from build123d import *

# Parameters (mm, degrees)
CUT_EXTRUDE_1_DEPTH = 8
SKETCH_7_R          = 4.1
CUT_EXTRUDE_3_DEPTH = 10


with BuildPart() as part:
    # 草图1 → 旋转1 (revolve)
    with BuildSketch(Plane.XY):
        Polygon((-9.5, 0), (9.5, 0), (9.5, 13), (8, 13), (8, 11.05), (-8, 11.05), (-8, 13), (-9.5, 13), align=None)
    revolve(axis=Axis((-9.5, 0, 0), (1, 0, 0)))

    # 草图2 → 切除-拉伸1 (cut, symmetric)
    with BuildSketch(Plane(origin=(0, 0, 0), x_dir=(0, 0, -1), z_dir=(1, 0, 0))):
        with BuildLine():
            Line((11.05, 0), (10, 0))
            ThreePointArc((10, 0), (9.969173337, 0.784590957), (9.876883406, 1.56434465))
            Line((9.876883406, 1.56434465), (10.913956164, 1.728600839))
            ThreePointArc((10.913956164, 1.728600839), (11.015936538, 0.866973008), (11.05, 0))
        make_face()
        with BuildLine():
            Line((10.509174505, -3.414637788), (9.510565163, -3.090169944))
            ThreePointArc((9.510565163, -3.090169944), (9.723699204, -2.334453639), (9.876883406, -1.56434465))
            Line((9.876883406, -1.56434465), (10.913956164, -1.728600839))
            ThreePointArc((10.913956164, -1.728600839), (10.74468762, -2.579571271), (10.509174505, -3.414637788))
        make_face()
        with BuildLine():
            Line((8.939637788, -6.495027038), (8.090169944, -5.877852523))
            ThreePointArc((8.090169944, -5.877852523), (8.526401644, -5.224985647), (8.910065242, -4.539904997))
            Line((8.910065242, -4.539904997), (9.845622092, -5.016595022))
            ThreePointArc((9.845622092, -5.016595022), (9.421673816, -5.77360914), (8.939637788, -6.495027038))
        make_face()
        with BuildLine():
            Line((6.495027038, -8.939637788), (5.877852523, -8.090169944))
            ThreePointArc((5.877852523, -8.090169944), (6.494480483, -7.604059656), (7.071067812, -7.071067812))
            Line((7.071067812, -7.071067812), (7.813529932, -7.813529932))
            ThreePointArc((7.813529932, -7.813529932), (7.176400934, -8.40248592), (6.495027038, -8.939637788))
        make_face()
        with BuildLine():
            Line((3.414637788, -10.509174505), (3.090169944, -9.510565163))
            ThreePointArc((3.090169944, -9.510565163), (3.826834324, -9.238795325), (4.539904997, -8.910065242))
            Line((4.539904997, -8.910065242), (5.016595022, -9.845622092))
            ThreePointArc((5.016595022, -9.845622092), (4.228651928, -10.208868834), (3.414637788, -10.509174505))
        make_face()
        with BuildLine():
            Line((0, -11.05), (0, -10))
            ThreePointArc((0, -10), (0.784590957, -9.969173337), (1.56434465, -9.876883406))
            Line((1.56434465, -9.876883406), (1.728600839, -10.913956164))
            ThreePointArc((1.728600839, -10.913956164), (0.866973008, -11.015936538), (0, -11.05))
        make_face()
        with BuildLine():
            Line((-3.414637788, -10.509174505), (-3.090169944, -9.510565163))
            ThreePointArc((-3.090169944, -9.510565163), (-2.334453639, -9.723699204), (-1.56434465, -9.876883406))
            Line((-1.56434465, -9.876883406), (-1.728600839, -10.913956164))
            ThreePointArc((-1.728600839, -10.913956164), (-2.579571271, -10.74468762), (-3.414637788, -10.509174505))
        make_face()
        with BuildLine():
            Line((-6.495027038, -8.939637788), (-5.877852523, -8.090169944))
            ThreePointArc((-5.877852523, -8.090169944), (-5.224985647, -8.526401644), (-4.539904997, -8.910065242))
            Line((-4.539904997, -8.910065242), (-5.016595022, -9.845622092))
            ThreePointArc((-5.016595022, -9.845622092), (-5.77360914, -9.421673816), (-6.495027038, -8.939637788))
        make_face()
        with BuildLine():
            Line((-8.939637788, -6.495027038), (-8.090169944, -5.877852523))
            ThreePointArc((-8.090169944, -5.877852523), (-7.604059656, -6.494480483), (-7.071067812, -7.071067812))
            Line((-7.071067812, -7.071067812), (-7.813529932, -7.813529932))
            ThreePointArc((-7.813529932, -7.813529932), (-8.40248592, -7.176400934), (-8.939637788, -6.495027038))
        make_face()
        with BuildLine():
            Line((-10.509174505, -3.414637788), (-9.510565163, -3.090169944))
            ThreePointArc((-9.510565163, -3.090169944), (-9.238795325, -3.826834324), (-8.910065242, -4.539904997))
            Line((-8.910065242, -4.539904997), (-9.845622092, -5.016595022))
            ThreePointArc((-9.845622092, -5.016595022), (-10.208868834, -4.228651928), (-10.509174505, -3.414637788))
        make_face()
        with BuildLine():
            Line((-11.05, 0), (-10, 0))
            ThreePointArc((-10, 0), (-9.969173337, -0.784590957), (-9.876883406, -1.56434465))
            Line((-9.876883406, -1.56434465), (-10.913956164, -1.728600839))
            ThreePointArc((-10.913956164, -1.728600839), (-11.015936538, -0.866973008), (-11.05, 0))
        make_face()
        with BuildLine():
            Line((-10.509174505, 3.414637788), (-9.510565163, 3.090169944))
            ThreePointArc((-9.510565163, 3.090169944), (-9.723699204, 2.334453639), (-9.876883406, 1.56434465))
            Line((-9.876883406, 1.56434465), (-10.913956164, 1.728600839))
            ThreePointArc((-10.913956164, 1.728600839), (-10.74468762, 2.579571271), (-10.509174505, 3.414637788))
        make_face()
        with BuildLine():
            Line((-8.939637788, 6.495027038), (-8.090169944, 5.877852523))
            ThreePointArc((-8.090169944, 5.877852523), (-8.526401644, 5.224985647), (-8.910065242, 4.539904997))
            Line((-8.910065242, 4.539904997), (-9.845622092, 5.016595022))
            ThreePointArc((-9.845622092, 5.016595022), (-9.421673816, 5.77360914), (-8.939637788, 6.495027038))
        make_face()
        with BuildLine():
            Line((-6.495027038, 8.939637788), (-5.877852523, 8.090169944))
            ThreePointArc((-5.877852523, 8.090169944), (-6.494480483, 7.604059656), (-7.071067812, 7.071067812))
            Line((-7.071067812, 7.071067812), (-7.813529932, 7.813529932))
            ThreePointArc((-7.813529932, 7.813529932), (-7.176400934, 8.40248592), (-6.495027038, 8.939637788))
        make_face()
        with BuildLine():
            Line((-3.414637788, 10.509174505), (-3.090169944, 9.510565163))
            ThreePointArc((-3.090169944, 9.510565163), (-3.826834324, 9.238795325), (-4.539904997, 8.910065242))
            Line((-4.539904997, 8.910065242), (-5.016595022, 9.845622092))
            ThreePointArc((-5.016595022, 9.845622092), (-4.228651928, 10.208868834), (-3.414637788, 10.509174505))
        make_face()
        with BuildLine():
            Line((0, 11.05), (0, 10))
            ThreePointArc((0, 10), (-0.784590957, 9.969173337), (-1.56434465, 9.876883406))
            Line((-1.56434465, 9.876883406), (-1.728600839, 10.913956164))
            ThreePointArc((-1.728600839, 10.913956164), (-0.866973008, 11.015936538), (0, 11.05))
        make_face()
        with BuildLine():
            Line((3.414637788, 10.509174505), (3.090169944, 9.510565163))
            ThreePointArc((3.090169944, 9.510565163), (2.334453639, 9.723699204), (1.56434465, 9.876883406))
            Line((1.56434465, 9.876883406), (1.728600839, 10.913956164))
            ThreePointArc((1.728600839, 10.913956164), (2.579571271, 10.74468762), (3.414637788, 10.509174505))
        make_face()
        with BuildLine():
            Line((6.495027038, 8.939637788), (5.877852523, 8.090169944))
            ThreePointArc((5.877852523, 8.090169944), (5.224985647, 8.526401644), (4.539904997, 8.910065242))
            Line((4.539904997, 8.910065242), (5.016595022, 9.845622092))
            ThreePointArc((5.016595022, 9.845622092), (5.77360914, 9.421673816), (6.495027038, 8.939637788))
        make_face()
        with BuildLine():
            Line((8.939637788, 6.495027038), (8.090169944, 5.877852523))
            ThreePointArc((8.090169944, 5.877852523), (7.604059656, 6.494480483), (7.071067812, 7.071067812))
            Line((7.071067812, 7.071067812), (7.813529932, 7.813529932))
            ThreePointArc((7.813529932, 7.813529932), (8.40248592, 7.176400934), (8.939637788, 6.495027038))
        make_face()
        with BuildLine():
            Line((10.509174505, 3.414637788), (9.510565163, 3.090169944))
            ThreePointArc((9.510565163, 3.090169944), (9.238795325, 3.826834324), (8.910065242, 4.539904997))
            Line((8.910065242, 4.539904997), (9.845622092, 5.016595022))
            ThreePointArc((9.845622092, 5.016595022), (10.208868834, 4.228651928), (10.509174505, 3.414637788))
        make_face()
    extrude(amount=CUT_EXTRUDE_1_DEPTH, both=True, mode=Mode.SUBTRACT)

    # 草图7 → 切除-拉伸3 (cut, symmetric)
    with BuildSketch(Plane(origin=(0, 0, 0), x_dir=(0, 0, -1), z_dir=(1, 0, 0))):
        Circle(SKETCH_7_R)
    extrude(amount=CUT_EXTRUDE_3_DEPTH, both=True, mode=Mode.SUBTRACT)


solid = part.part
Geometry check sheet. Reference: the model listing, model coordinates, mm. A direction names the side the tool comes from. Round coordinates to 2 decimals unless told otherwise and drop trailing zeros. Write each loop counter-clockwise with the first axis right and the second up, starting at its lowest first coordinate (ties: lowest second). Pieces come first, ordered by that corner, then holes. Notation, with made-up numbers: (81.5, 14) -> (133.5, 14) arc R14 ccw to (133.5, 18) -> close; hole circle Ø1 at (-28.75, 55.5). An arc over 180 degrees is marked (long way). One line per item, written item: value. Start each with the question number.
(1) Draft check along Y on faces 1 (the flat face through (-9.5, -3.1, 3.1)), 2 (the cylindrical face through (-0.112, -0.879, -11.015)), 3 (the cylindrical face through (0.133, 4.065, 0.534)). Enter one of: +Y half, -Y half, draft (parallel to the pull), parting line (faces both ways), or undercut.
(2) Go/stop test with flat-tipped pins: pin 1 Ø8 at (x, y) = (-1.5, 3.5) entering from -Z; pin 2 Ø0.8 at (x, y) = (-1.5, -10.5) entering from -Z; pin 3 Ø0.8 at (x, y) = (-1.5, 10.5) entering from +Z; pin 4 Ø12 at (y, z) = (0.5, 1.5) entering from +X. Record where each tip stops, or that it passes through.
(3) Access from +Z, -Z, +X, -X, +Y, -Y to the whole of each face (thin tool, end or side, straight path). Record for faces 4 (the flat face through (-8, 3, 10)), 5 (the flat face through (-0.1, 0, -10.5)), 6 (the cylindrical face through (-0.112, -2.568, 10.748)).
(4) Cross-section at A-A, the plane y = -0.5. Record the cut outline in (x, z).
(5) Scan lines: line 1 (X direction, y = 11.5, z = -2); line 2 (Z direction, x = 0.75, y = -3.75); line 3 (Z direction, x = -1, y = 7.5). Record each from-to range of solid material in increasing order. Write a range as [from, to].
Answer:
1. face 1: draft
1. face 2: -Y half
1. face 3: undercut
2. pin 1: z = -11.05
2. pin 2: z = -3.41
2. pin 3: z = 3.41
2. pin 4: x = 9.5
3. face 4: none
3. face 5: -Z
3. face 6: +Z, -Y
4. outline: (-9.5, -12.99) -> (-8, -12.99) -> (-8, -11.04) -> (8, -11.04) -> (8, -12.99) -> (9.5, -12.99) -> (9.5, -4.07) -> (-9.5, -4.07) -> close; (-9.5, 4.07) -> (9.5, 4.07) -> (9.5, 12.99) -> (8, 12.99) -> (8, 9.99) -> (-8, 9.99) -> (-8, 12.99) -> (-9.5, 12.99) -> close
5. line 1: [-9.5, -8], [8, 9.5]
5. line 2: [-10.39, -1.66], [1.66, 9.27]
5. line 3: [-7.5, 6.61], [7.5, 8.11]
